Part print with two shaded views. Sizes in mm from the minimum x, y, z corner. Coordinates: 2 decimals unless noted, no trailing zeros. Write each loop counter-clockwise with the first axis right and the second up, starting at its lowest first coordinate (ties: lowest second). Pieces come first, ordered by that corner, then holes. Notation, with made-up numbers: M 74.25,17 L 112.25,17 A21 ccw 112.25,49 Z; hole C 72.5,55.5 d11. An arc over 180 degrees is marked long. One line per question, with ' | ' between items. Start each with the question number.
(1) Cut at A-A (x = 12.7). Write the cut outline in (y, z).
(2) Cut at D-D (x = 38.5). Write the cut outline in (y, z) (1 decimal).
(3) Cut at B-B (z = 12.7). Write the cut outline in (x, y).
(4) Wall check: probe 1 along X at (y, z) = (1.4, 12.7); probe 2 along Z at (x, y) = (12.7, 1.7); probe 3 along X at (y, z) = (0.45, 14) (1 decimal). Give the ranges that are in metal, low to high.
(5) Two-plate mould, pull along Z, no slides. Class the marked faces 1, 2, 3 and 4: +Z half, -Z half, draft (parallel to the pull), parting line (faces both ways), or undercut.
(6) Cut at C-C (y = 2.5). Count the separate pieces of the cut face and the enclosed holes in it, plus the area to 3 significant figures.
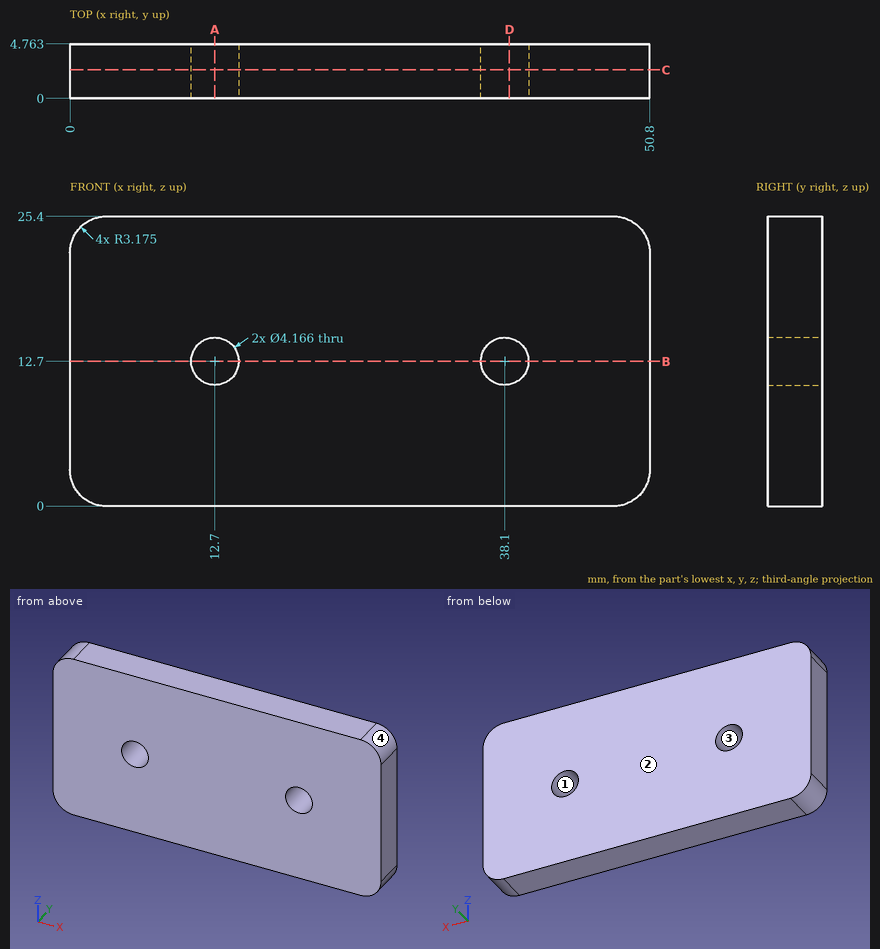
Filled in:
1) outline: M 0,0 L 4.76,0 L 4.76,10.62 L 0,10.62 Z; M 0,14.78 L 4.76,14.78 L 4.76,25.4 L 0,25.4 Z
2) outline: M 0,0 L 4.8,0 L 4.8,10.7 L 0,10.7 Z; M 0,14.7 L 4.8,14.7 L 4.8,25.4 L 0,25.4 Z
3) outline: M 0,0 L 10.62,0 L 10.62,4.76 L 0,4.76 Z; M 14.78,0 L 36.02,0 L 36.02,4.76 L 14.78,4.76 Z; M 40.18,0 L 50.8,0 L 50.8,4.76 L 40.18,4.76 Z
4) probe 1: 0 to 10.62, 14.78 to 36.02, 40.18 to 50.8 | probe 2: 0 to 10.62, 14.78 to 25.4 | probe 3: 0 to 11.1, 14.3 to 36.5, 39.7 to 50.8
5) face 1: undercut | face 2: draft | face 3: undercut | face 4: +Z half
6) separate pieces: 1 | enclosed holes: 2 | area: 1,250 mm²
